Could you check a few things on this model? Use its own coordinates, in mm. A direction names the side the tool comes from. Give positions to 0.01 mm unless a question says otherwise; leave off trailing zeros. Loops run counter-clockwise (first coordinate to the right, second up) from the corner with the lowest first, then second, coordinate; pieces in that order, holes last.
1. Thinking about a two-plate mould opening in Y: for faces 1 (the flat face through (16, -16, -12)), 2 (the conical face through (15.45, 15.29, 1.38)), 3 (the flat face through (-18, 18, 4)), which applies, +Y half, -Y half, draft (parallel to the pull), parting line (faces both ways), or undercut?
2. Imagine slicing it at A-A (x = 0). List the corners of the cut face in (y, z) for me, plus the area to 3 significant figures.
3. I need wall thicknesses on line 1 along Y through (x, z) = (15.5, 5.55); line 2 along Y through (x, z) = (15, 6). Which ranges of each line are inside material? Lowest first, please.
4. For faces 4 (the cylindrical face through (-14.579, 16.345, 4.958)), 5 (the cylindrical face through (20.844, -14.947, -28.056)), which set-ups out of +Z, -Z, +X, -X, +Y, -Y let a thin tool reach every point of the face, with its end or its side?
5. Imagine slicing it at B-B (z = -21.5). List the corners of the cut face in (x, y) for me.
6. Imagine slicing it at C-C (y = 18.5). List the corners of the cut face in (x, z) for me.
7. For P1, Ø2, axis at x = -9.5, z = -20, coming from the +Y side; P2, Ø17, axis at x = 4.5, z = -13.5, coming from the -Y side; P3, Ø1.5, axis at x = -7, z = 9, coming from the +Y side; P4, Ø21, axis at x = -4, y = -8.5, coming from the +Z side, each with a flat end and sliding along its axis, tell me the tip position at first contact or that it passes through.
8. Imagine slicing it at D-D (x = 17.5). List the corners of the cut face in (y, z) for me, plus the area to 3 significant figures.
```python
from build123d import *

# Parameters (mm, degrees)
EXTRUDE_START               = -40
EXTRUDE_2_DEPTH             = 40
EXTRUDE_START_2             = -8
EXTRUDE_2_2_DEPTH           = 8
EXTRUDE_2_3_DEPTH           = 8
EXTRUDE_2_4_OUTLINE_R       = 2.5
EXTRUDE_2_4_DEPTH           = 20.5
FILLET_1_R                  = 2
HOLE_WIZARD_2_5_2_5_1_D     = 2.5
HOLE_WIZARD_2_5_2_5_1_DEPTH = 6
HOLE_WIZARD_2_5_2_5_1_TIP   = 0.751075774
HOLE_WIZARD_2_5_2_5_2_D     = 2.5
HOLE_WIZARD_2_5_2_5_2_DEPTH = 6
HOLE_WIZARD_2_5_2_5_2_TIP   = 0.751075774
HOLE_WIZARD_2_5_2_5_3_D     = 2.5
HOLE_WIZARD_2_5_2_5_3_DEPTH = 6
HOLE_WIZARD_2_5_2_5_3_TIP   = 0.751075774
HOLE_WIZARD_2_5_2_5_4_D     = 2.5
HOLE_WIZARD_2_5_2_5_4_DEPTH = 6
HOLE_WIZARD_2_5_2_5_4_TIP   = 0.751075774
SKETCH_15_R                 = 11
SKETCH_15_R_2               = 2
EXTRUDE_3_DEPTH             = 1.5


with BuildPart() as part:
    # Бобышка-Вытянуть2: read off the stored shape, not the designer's step
    # Бобышка-Вытянуть2 outline → Бобышка-Вытянуть2 (new body)
    with BuildSketch(Plane.XY.offset(8).offset(EXTRUDE_START)):
        with BuildLine():
            ThreePointArc((19.828427125, -12.171572875), (20.366719307, -11.503053413), (20.75, -10.735086841))
            Line((20.75, -10.735086841), (20.75, 10.735086841))
            ThreePointArc((20.75, 10.735086841), (20.366719307, 11.503053413), (19.828427125, 12.171572875))
            Line((19.828427125, 12.171572875), (12.171572875, 19.828427125))
            ThreePointArc((12.171572875, 19.828427125), (11.503053413, 20.366719307), (10.735086841, 20.75))
            Line((10.735086841, 20.75), (-10.735086841, 20.75))
            ThreePointArc((-10.735086841, 20.75), (-11.503053413, 20.366719307), (-12.171572875, 19.828427125))
            Line((-12.171572875, 19.828427125), (-19.828427125, 12.171572875))
            ThreePointArc((-19.828427125, 12.171572875), (-20.366719307, 11.503053413), (-20.75, 10.735086841))
            Line((-20.75, 10.735086841), (-20.75, -10.735086841))
            ThreePointArc((-20.75, -10.735086841), (-20.366719307, -11.503053413), (-19.828427125, -12.171572875))
            Line((-19.828427125, -12.171572875), (-12.171572875, -19.828427125))
            ThreePointArc((-12.171572875, -19.828427125), (-11.503053413, -20.366719307), (-10.735086841, -20.75))
            Line((-10.735086841, -20.75), (10.735086841, -20.75))
            ThreePointArc((10.735086841, -20.75), (11.503053413, -20.366719307), (12.171572875, -19.828427125))
            Line((12.171572875, -19.828427125), (19.828427125, -12.171572875))
        make_face()
    extrude(amount=EXTRUDE_2_DEPTH)

    # Extrude 2 2 outline → Extrude 2 2 (add)
    with BuildSketch(Plane.XY.offset(8).offset(EXTRUDE_START_2)):
        Polygon((21, 15), (15, 21), (-15, 21), (-21, 15), (-21, -15), (-15, -21), (15, -21), (21, -15), align=None)
        with BuildLine():
            ThreePointArc((20.75, -10.735086841), (20.366719307, -11.503053413), (19.828427125, -12.171572875))
            Line((19.828427125, -12.171572875), (12.171572875, -19.828427125))
            ThreePointArc((12.171572875, -19.828427125), (11.503053413, -20.366719307), (10.735086841, -20.75))
            Line((10.735086841, -20.75), (-10.735086841, -20.75))
            ThreePointArc((-10.735086841, -20.75), (-11.503053413, -20.366719307), (-12.171572875, -19.828427125))
            Line((-12.171572875, -19.828427125), (-19.828427125, -12.171572875))
            ThreePointArc((-19.828427125, -12.171572875), (-20.366719307, -11.503053413), (-20.75, -10.735086841))
            Line((-20.75, -10.735086841), (-20.75, 10.735086841))
            ThreePointArc((-20.75, 10.735086841), (-20.366719307, 11.503053413), (-19.828427125, 12.171572875))
            Line((-19.828427125, 12.171572875), (-12.171572875, 19.828427125))
            ThreePointArc((-12.171572875, 19.828427125), (-11.503053413, 20.366719307), (-10.735086841, 20.75))
            Line((-10.735086841, 20.75), (10.735086841, 20.75))
            ThreePointArc((10.735086841, 20.75), (11.503053413, 20.366719307), (12.171572875, 19.828427125))
            Line((12.171572875, 19.828427125), (19.828427125, 12.171572875))
            ThreePointArc((19.828427125, 12.171572875), (20.366719307, 11.503053413), (20.75, 10.735086841))
            Line((20.75, 10.735086841), (20.75, -10.735086841))
        make_face(mode=Mode.SUBTRACT)
    extrude(amount=EXTRUDE_2_2_DEPTH)

    # Extrude 2 3 outline → Extrude 2 3 (add)
    with BuildSketch(Plane.XY.offset(8).offset(EXTRUDE_START)):
        with BuildLine():
            Line((21, -14.171572875), (21, 14.171572875))
            ThreePointArc((21, 14.171572875), (20.847759065, 14.93693974), (20.414213562, 15.585786438))
            Line((20.414213562, 15.585786438), (15.585786438, 20.414213562))
            ThreePointArc((15.585786438, 20.414213562), (14.93693974, 20.847759065), (14.171572875, 21))
            Line((14.171572875, 21), (-14.171572875, 21))
            ThreePointArc((-14.171572875, 21), (-14.93693974, 20.847759065), (-15.585786438, 20.414213562))
            Line((-15.585786438, 20.414213562), (-20.414213562, 15.585786438))
            ThreePointArc((-20.414213562, 15.585786438), (-20.847759065, 14.93693974), (-21, 14.171572875))
            Line((-21, 14.171572875), (-21, -14.171572875))
            ThreePointArc((-21, -14.171572875), (-20.847759065, -14.93693974), (-20.414213562, -15.585786438))
            Line((-20.414213562, -15.585786438), (-15.585786438, -20.414213562))
            ThreePointArc((-15.585786438, -20.414213562), (-14.93693974, -20.847759065), (-14.171572875, -21))
            Line((-14.171572875, -21), (14.171572875, -21))
            ThreePointArc((14.171572875, -21), (14.93693974, -20.847759065), (15.585786438, -20.414213562))
            Line((15.585786438, -20.414213562), (20.414213562, -15.585786438))
            ThreePointArc((20.414213562, -15.585786438), (20.847759065, -14.93693974), (21, -14.171572875))
        make_face()
        with BuildLine():
            Line((20.75, 10.735086841), (20.75, -10.735086841))
            ThreePointArc((20.75, -10.735086841), (20.366719307, -11.503053413), (19.828427125, -12.171572875))
            Line((19.828427125, -12.171572875), (12.171572875, -19.828427125))
            ThreePointArc((12.171572875, -19.828427125), (11.503053413, -20.366719307), (10.735086841, -20.75))
            Line((10.735086841, -20.75), (-10.735086841, -20.75))
            ThreePointArc((-10.735086841, -20.75), (-11.503053413, -20.366719307), (-12.171572875, -19.828427125))
            Line((-12.171572875, -19.828427125), (-19.828427125, -12.171572875))
            ThreePointArc((-19.828427125, -12.171572875), (-20.366719307, -11.503053413), (-20.75, -10.735086841))
            Line((-20.75, -10.735086841), (-20.75, 10.735086841))
            ThreePointArc((-20.75, 10.735086841), (-20.366719307, 11.503053413), (-19.828427125, 12.171572875))
            Line((-19.828427125, 12.171572875), (-12.171572875, 19.828427125))
            ThreePointArc((-12.171572875, 19.828427125), (-11.503053413, 20.366719307), (-10.735086841, 20.75))
            Line((-10.735086841, 20.75), (10.735086841, 20.75))
            ThreePointArc((10.735086841, 20.75), (11.503053413, 20.366719307), (12.171572875, 19.828427125))
            Line((12.171572875, 19.828427125), (19.828427125, 12.171572875))
            ThreePointArc((19.828427125, 12.171572875), (20.366719307, 11.503053413), (20.75, 10.735086841))
        make_face(mode=Mode.SUBTRACT)
    extrude(amount=EXTRUDE_2_3_DEPTH)

    # Extrude 2 4 outline → Extrude 2 4 (add)
    with BuildSketch(Plane.XY.offset(8)):
        Circle(EXTRUDE_2_4_OUTLINE_R)
    extrude(amount=EXTRUDE_2_4_DEPTH)

    # Скругление1
    fillet_1_edges = [part.edges().sort_by_distance(p)[0] for p in [
        (15, -21, 4),
        (-15, -21, 4),
        (-21, -15, 4),
        (15, 21, 4),
        (21, -15, 4),
        (-15, 21, 4),
        (21, 15, 4),
        (-21, 15, 4),
    ]]
    fillet(fillet_1_edges, radius=FILLET_1_R)

    # Диаметр отверстия Ø2.5 (2.5)1
    with Locations(Plane.XY.offset(8)):
        with Locations((-15.5, 15.5)):
            Hole(HOLE_WIZARD_2_5_2_5_1_D / 2, depth=HOLE_WIZARD_2_5_2_5_1_DEPTH)
            with Locations((0, 0, -(HOLE_WIZARD_2_5_2_5_1_DEPTH + HOLE_WIZARD_2_5_2_5_1_TIP / 2))):  # 118° drill point
                Cone(0, HOLE_WIZARD_2_5_2_5_1_D / 2, HOLE_WIZARD_2_5_2_5_1_TIP, mode=Mode.SUBTRACT)

    # Диаметр отверстия Ø2.5 (2.5)2
    with Locations(Plane.XY.offset(8)):
        with Locations((15.5, 15.5)):
            Hole(HOLE_WIZARD_2_5_2_5_2_D / 2, depth=HOLE_WIZARD_2_5_2_5_2_DEPTH)
            with Locations((0, 0, -(HOLE_WIZARD_2_5_2_5_2_DEPTH + HOLE_WIZARD_2_5_2_5_2_TIP / 2))):  # 118° drill point
                Cone(0, HOLE_WIZARD_2_5_2_5_2_D / 2, HOLE_WIZARD_2_5_2_5_2_TIP, mode=Mode.SUBTRACT)

    # Диаметр отверстия Ø2.5 (2.5)3
    with Locations(Plane.XY.offset(8)):
        with Locations((-15.5, -15.5)):
            Hole(HOLE_WIZARD_2_5_2_5_3_D / 2, depth=HOLE_WIZARD_2_5_2_5_3_DEPTH)
            with Locations((0, 0, -(HOLE_WIZARD_2_5_2_5_3_DEPTH + HOLE_WIZARD_2_5_2_5_3_TIP / 2))):  # 118° drill point
                Cone(0, HOLE_WIZARD_2_5_2_5_3_D / 2, HOLE_WIZARD_2_5_2_5_3_TIP, mode=Mode.SUBTRACT)

    # Диаметр отверстия Ø2.5 (2.5)4
    with Locations(Plane.XY.offset(8)):
        with Locations((15.5, -15.5)):
            Hole(HOLE_WIZARD_2_5_2_5_4_D / 2, depth=HOLE_WIZARD_2_5_2_5_4_DEPTH)
            with Locations((0, 0, -(HOLE_WIZARD_2_5_2_5_4_DEPTH + HOLE_WIZARD_2_5_2_5_4_TIP / 2))):  # 118° drill point
                Cone(0, HOLE_WIZARD_2_5_2_5_4_D / 2, HOLE_WIZARD_2_5_2_5_4_TIP, mode=Mode.SUBTRACT)

    # Эскиз15 → Бобышка-Вытянуть3 (add)
    with BuildSketch(Plane.XY.offset(8)):
        Circle(SKETCH_15_R)
        Circle(SKETCH_15_R_2, mode=Mode.SUBTRACT)
    extrude(amount=EXTRUDE_3_DEPTH)


solid = part.part
```
Derived:
1. face 1: -Y half
1. face 2: undercut
1. face 3: +Y half
2. outline: (-21, -32) - (21, -32) - (21, -24) - (20.75, -24) - (20.75, 0) - (21, 0) - (21, 8) - (11, 8) - (11, 9.5) - (2.5, 9.5) - (2.5, 28.5) - (-2.5, 28.5) - (-2.5, 9.5) - (-11, 9.5) - (-11, 8) - (-21, 8) - (-21, 0) - (-20.75, 0) - (-20.75, -24) - (-21, -24) - close
2. area: 1,800 mm2
3. line 1: y = -20.5 to -16.75, -14.25 to 14.25, 16.75 to 20.5
3. line 2: y = -20.82 to -16.65, -14.35 to 14.35, 16.65 to 20.82
4. face 4: +Z
4. face 5: +Z, -Z, +X, -Y
5. outline: (-20.75, -10.74) arc R4 ccw to (-19.83, -12.17) - (-12.17, -19.83) arc R4 ccw to (-10.74, -20.75) - (10.74, -20.75) arc R4 ccw to (12.17, -19.83) - (19.83, -12.17) arc R4 ccw to (20.75, -10.74) - (20.75, 10.74) arc R4 ccw to (19.83, 12.17) - (12.17, 19.83) arc R4 ccw to (10.74, 20.75) - (-10.74, 20.75) arc R4 ccw to (-12.17, 19.83) - (-19.83, 12.17) arc R4 ccw to (-20.75, 10.74) - close
6. outline: (-17.5, -32) - (17.5, -32) - (17.5, -24) - (13.5, -24) - (13.5, 0) - (17.5, 0) - (17.5, 8) - (-17.5, 8) - (-17.5, 0) - (-13.5, 0) - (-13.5, -24) - (-17.5, -24) - close
7. P1: stops at y = 20.75
7. P2: stops at y = -20.75
7. P3: stops at y = 9.05
7. P4: stops at z = 28.5
8. outline: (-18.5, -32) - (18.5, -32) - (18.5, -24) - (14.5, -24) - (14.5, 0) - (18.5, 0) - (18.5, 8) - (-18.5, 8) - (-18.5, 0) - (-14.5, 0) - (-14.5, -24) - (-18.5, -24) - close
8. area: 1,290 mm2
